```python
from build123d import *

# Parameters (mm, degrees)
PAD_DEPTH         = 4
POCKET_DEPTH      = 0.5
SKETCH002_R       = 4.75
PAD001_DEPTH      = 1.2
PAD001_DEPTH_BACK = 16.7
SKETCH003_R       = 4
PAD002_DEPTH      = 7.5
SKETCH004_R       = 1.95
POCKET001_DEPTH   = 61.83559
SKETCH005_R       = 1
POCKET002_DEPTH   = 52.001
FILLET_R          = 1
FILLET001_R       = 1
FILLET002_R       = 1


with BuildPart() as part:
    # Sketch → Pad (new body)
    with BuildSketch(Plane(origin=(-43, 85, 6), x_dir=(-1, 0, 0), z_dir=(0, -1, 0))):
        Polygon((-25, -15.5), (-25, -8), (-10, -8), (-10, -0.5), (12, -0.25447), (71, 34), (92, -60), (88, -60), (62, 13), (10, -15.5), align=None)
    extrude(amount=PAD_DEPTH)

    # Sketch001 → Pocket (cut)
    with BuildSketch(Plane(origin=(-43, 81, 6), x_dir=(-1, 0, 0), z_dir=(0, -1, 0))):
        with BuildLine():
            Line((23.5, -1.5), (23.5, 1.5))
            ThreePointArc((24.213026, 2.776977), (23.690332, 2.231279), (23.5, 1.5))
            Line((24.213026, 2.776977), (67.213026, 29.276977))
            ThreePointArc((69.45638, 28.359107), (68.56802, 29.388291), (67.213026, 29.276977))
            Line((69.45638, 28.359107), (87.45638, -44.640893))
            ThreePointArc((84.575842, -45.470927), (86.41533, -46.441354), (87.45638, -44.640893))
            Line((84.575842, -45.470927), (64.424158, 15.470927))
            ThreePointArc((64.424158, 15.470927), (63.562865, 16.390389), (62.304506, 16.329017))
            Line((62.304506, 16.329017), (25.695494, -2.829017))
            ThreePointArc((23.5, -1.5), (24.223225, -2.783207), (25.695494, -2.829017))
        make_face()
    extrude(amount=-POCKET_DEPTH, mode=Mode.SUBTRACT)

    # Sketch002 → Pad001 (new body, two sides)
    with BuildSketch(Plane(origin=(-43.004334, 85, 6.388347), x_dir=(0.999938, 0, 0.01116), z_dir=(0.01116, 0, -0.999938))) as pad001_sk:
        with Locations((0, 2)):
            Circle(SKETCH002_R)
    extrude(amount=PAD001_DEPTH)
    extrude(pad001_sk.sketch, amount=-PAD001_DEPTH_BACK)

    # Sketch003 → Pad002 (new body)
    with BuildSketch(Plane(origin=(-43, 85, 14), x_dir=(1, 0, 0), z_dir=(0, 0, -1))):
        with Locations((20, 2)):
            Circle(SKETCH003_R)
    extrude(amount=-PAD002_DEPTH)

    # Sketch004 → Pocket001 (cut, through all)
    with BuildSketch(Plane(origin=(-42.990942, 85, 5.188422), x_dir=(0.999938, 0, 0.01116), z_dir=(0.01116, 0, -0.999938))):
        with Locations((0, 2)):
            Circle(SKETCH004_R)
    extrude(amount=-POCKET001_DEPTH, mode=Mode.SUBTRACT)

    # Sketch005 → Pocket002 (cut, through all)
    with BuildSketch(Plane(origin=(-43, 85, 14), x_dir=(1, 0, 0), z_dir=(0, 0, -1))):
        with Locations((20, 2)):
            Circle(SKETCH005_R)
    extrude(amount=-POCKET002_DEPTH, mode=Mode.SUBTRACT)

    # Fillet
    fillet_edges = [part.edges().sort_by_distance(p)[0] for p in [
        (-18, 85, 17.75),
    ]]
    fillet(fillet_edges, radius=FILLET_R)

    # Fillet001
    fillet001_edges = [part.edges().sort_by_distance(p)[0] for p in [
        (-18, 81, 17.75),
    ]]
    fillet(fillet001_edges, radius=FILLET001_R)

    # Fillet002
    fillet002_edges = [part.edges().sort_by_distance(p)[0] for p in [
        (-33, 83, 6.5),
    ]]
    fillet(fillet002_edges, radius=FILLET002_R)


solid = part.part
```
CAD build for the part. Positions are in the model's coordinates, mm. A direction names the side the tool comes from. Coordinates: 2 decimals unless noted, no trailing zeros. Loops run counter-clockwise (first coordinate to the right, second up) from the corner with the lowest first, then second, coordinate; pieces in that order, holes last. Notation, with made-up numbers: (74.25, 63.25) - (99.25, 63.25) arc R8 cw to (99.25, 74.25) - close; hole circle Ø11 at (3.5, 73.5). An arc over 180 degrees is marked (long way). Return JSON: item names as keys, results as strings.
1. Band-saw the part on B-B (x = -95.5). Give the cut face in (y, z).
Result:
{"outline": "(81, -17.26) - (85, -17.26) - (85, -1.79) - (81, -1.79) - (81, -5.2) - (81.5, -5.2) - (81.5, -14.21) - (81, -14.21) - close"}
2. Band-saw the part on D-D (x = -29). Give the cut face in (y, z).
Result:
{"outline": "(81, 14) - (85, 14) - (85, 21.5) - (81, 21.5) - close"}
3. 3-axis set-ups, long thin cutter, end or side, ignore diameter. For faces 1 (the cylindrical face through (-43.343, 81.067, 14.01)), 2 (the flat face through (-79.364, 83.028, 7.051)), 3 (the flat face through (-113, 81.5, 3)), 4 (the flat face through (-124.353, 83.028, 18.342)), 5 (the flat face through (-133, 83, 66)): which of +Z, -Z, +X, -X, +Y, -Y reach the whole face in a straight line?
Result:
{"face 1": "none", "face 2": "+Z, +Y, -Y", "face 3": "-Y", "face 4": "-Z, -X, +Y, -Y", "face 5": "+Z, +X, -X, +Y, -Y"}
4. Drop flat-ended pins along their axis: pin 1 (1.2 mm diameter, centred on x = -29.5, y = 82, fed in from -Z); pin 2 (5 mm diameter, centred on x = -96.5, y = 85, fed in from -Z); pin 3 (6 mm diameter, centred on x = -35, z = 14.5, fed in from -Y); pin 4 (1.8 mm diameter, centred on x = -23, y = 83, fed in from -Z). Give the stop position or say it passes through.
Result:
{"pin 1": "stops at z = 14", "pin 2": "stops at z = -19.29", "pin 3": "stops at y = 81", "pin 4": "passes through"}
5. Probe L1, parallel to X at y = 83, z = 16.5; L2, parallel to X at y = 83, z = 18.75; L3, parallel to Y at x = -70.5, z = 0.5. List the from-to ranges inside material, lowest first. Write a range as from..to.
Result:
{"L1": "x = -123.94..-113.37, -62.12..-45.07, -41.17..-24, -22..-18", "L2": "x = -124.44..-114.17, -58.02..-45.09, -41.19..-24, -22..-18", "L3": "y = 81..85"}
6. Mould opens along Z. For faces 6 (the flat face through (-117.641, 81.246, 21.427)), 7 (the flat face through (-88.41, 81.25, -9.84)), 8 (the flat face through (-33, 83, 11)), 9 (the flat face through (-118.18, 83.03, 30.01)) say: released by +Z, released by -Z, zero draft, split by the parting line, or undercut.
Result:
{"face 6": "undercut", "face 7": "undercut", "face 8": "zero draft", "face 9": "released by +Z"}
7. Band-saw the part on A-A (z = 27). Give the cut face in (x, y), and give its area (3 significant figures).
Result:
{"outline": "(-126.29, 81) - (-124.63, 81) - (-124.63, 81.5) - (-119.48, 81.5) - (-119.48, 81) - (-117.11, 81) - (-117.11, 85) - (-126.29, 85) - close", "area": "34.1 mm2"}
8. Band-saw the part on C-C (z = 11.5). State how many separate pieces and enclosed holes the cut face has, and give its area (3 significant figures).
Result:
{"separate pieces": "2", "enclosed holes": "1", "area": "217 mm2"}
